Could you check a few things on this drawing? It's one solid part, dimensions in mm from its lowest x, y, z. Give positions to 0.01 mm unless a question says otherwise; leave off trailing zeros. Loops run counter-clockwise (first coordinate to the right, second up) from the corner with the lowest first, then second, coordinate; pieces in that order, holes last. Notation, with made-up numbers: M 38.25,46.5 L 77.25,46.5 A35 cw 77.25,83.5 Z; hole C -16,46.25 d10. An arc over 180 degrees is marked long. Return JSON: item names as keys, results as strings. Group by question number.
1. If we section it at C-C (y = 11): Write out the boundary of the cut face in (x, z).
2. If we section it at D-D (y = 2.75): Write out the boundary of the cut face in (x, z).
3. Please list where these lines run through material, in increasing order: line 1 (X direction, y = 10.75, z = 0.85); line 2 (Y direction, x = 20.5, z = 4.7); line 3 (X direction, y = 18.25, z = 2.5).
4. If we section it at B-B (z = 4.1): Write out the boundary of the cut face in (x, y), plus the area to 3 significant figures.
5. If we section it at A-A (x = 20): Write out the boundary of the cut face in (y, z).
6. For pin 1 (1.5 mm diameter, centred on y = 6.5, z = 2, fed in from -X), with a flat end and sliding along its axis, tell me the tip position at first contact or that it passes through.
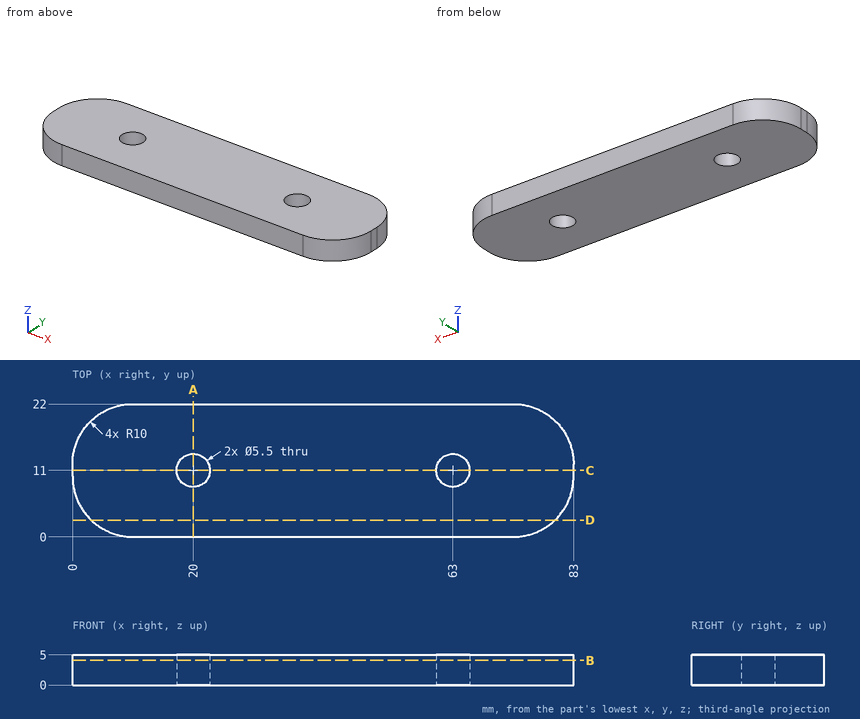
Answer:
{
 "1": {"outline": "M 0,0 L 17.25,0 L 17.25,5 L 0,5 Z; M 22.75,0 L 60.25,0 L 60.25,5 L 22.75,5 Z; M 65.75,0 L 83,0 L 83,5 L 65.75,5 Z"},
 "2": {"outline": "M 3.11,0 L 79.89,0 L 79.89,5 L 3.11,5 Z"},
 "3": {"line 1": "x = 0 to 17.26, 22.74 to 60.26, 65.74 to 83", "line 2": "y = 0 to 8.3, 13.7 to 22", "line 3": "x = 2.19 to 80.81"},
 "4": {"outline": "M 0,10 A10 ccw 10,0 L 73,0 A10 ccw 83,10 L 83,12 A10 ccw 73,22 L 10,22 A10 ccw 0,12 Z; hole C 20,11 d5.5; hole C 63,11 d5.5", "area": "1,690 mm²"},
 "5": {"outline": "M 0,0 L 8.25,0 L 8.25,5 L 0,5 Z; M 13.75,0 L 22,0 L 22,5 L 13.75,5 Z"},
 "6": {"pin 1": "stops at x = 0.39"}
}
